from build123d import *

# Parameters (mm, degrees)
BOSS_EXTRUDE1_DEPTH           = 2.5
SKETCH2_W                     = 7
SKETCH2_H                     = 2.5
BOSS_EXTRUDE2_DEPTH           = 9.5
CUT_EXTRUDE1_DEPTH            = 9.5
SKETCH4_R                     = 1.275
CUT_EXTRUDE2_DEPTH            = 9.5
CBORE_FOR_M2_SHCS1_AT_2_COUNT = 2
CBORE_FOR_M2_SHCS1_AT_2_PITCH = 10
SKETCH8_R                     = 2.2
CUT_EXTRUDE3_DEPTH            = 9.5
SKETCH11_W                    = 19.05
SKETCH11_H                    = 19.05
BOSS_EXTRUDE3_DEPTH           = 5
FILLET1_R                     = 0.2


with BuildPart() as part:
    # Sketch1 → Boss-Extrude1 (new body, symmetric)
    with BuildSketch(Plane(origin=(0, 0, 0), x_dir=(1, 0, 0), z_dir=(0, 1, 0))):
        with BuildLine():
            Line((1.96, 0), (8, 0))
            ThreePointArc((8, 0), (0, -8), (-8, 0))
            Line((-8, 0), (-1.96, 0))
            ThreePointArc((-1.96, 0), (0, -1.96), (1.96, 0))
        make_face()
    extrude(amount=BOSS_EXTRUDE1_DEPTH, both=True)

    # Sketch2 → Boss-Extrude2 (add)
    with BuildSketch(Plane(origin=(0, 2.5, 0), x_dir=(1, 0, 0), z_dir=(0, 1, 0))):
        with Locations((0, -5)):
            Rectangle(SKETCH2_W, SKETCH2_H)
    extrude(amount=BOSS_EXTRUDE2_DEPTH)

    # Sketch3 → Cut-Extrude1 (cut)
    with BuildSketch(Plane(origin=(0, 0, 3.75), x_dir=(-1, 0, 0), z_dir=(0, 0, -1))):
        with BuildLine():
            Line((-3.5, 8.5), (-3.5, 14.886359519))
            Line((-3.5, 14.886359519), (0, 16.809201746))
            Line((0, 16.809201746), (3.5, 14.5))
            Line((3.5, 14.5), (3.5, 8.5))
            ThreePointArc((3.5, 8.5), (0, 12), (-3.5, 8.5))
        make_face()
    extrude(amount=-CUT_EXTRUDE1_DEPTH, mode=Mode.SUBTRACT)

    # Sketch4 → Cut-Extrude2 (cut)
    with BuildSketch(Plane(origin=(0, 0, 3.75), x_dir=(-1, 0, 0), z_dir=(0, 0, -1))):
        with Locations((0, 8.5)):
            Circle(SKETCH4_R)
    extrude(amount=-CUT_EXTRUDE2_DEPTH, mode=Mode.SUBTRACT)

    # Sketch7 → CBORE for M2 SHCS1 (revolve, cut)
    with BuildSketch(Plane(origin=(5, 0, 7), x_dir=(0, -1, 0), z_dir=(1, 0, 0))):
        Polygon((0, 0), (0, 7), (1.2, 7), (1.2, 2), (2.2, 2), (2.2, 0), align=None)
    cbore_for_m2_shcs1 = revolve(axis=Axis((5, 0, 13.35), (0, 0, -1)), mode=Mode.SUBTRACT)

    # CBORE for M2 SHCS1 at 2: CBORE for M2 SHCS1 ×2
    with Locations(*[(-i * CBORE_FOR_M2_SHCS1_AT_2_PITCH, 0, 0) for i in range(1, CBORE_FOR_M2_SHCS1_AT_2_COUNT)]):
        add(cbore_for_m2_shcs1, mode=Mode.SUBTRACT)

    # Sketch8 → Cut-Extrude3 (cut)
    with BuildSketch(Plane(origin=(0, 0, 7), x_dir=(-1, 0, 0), z_dir=(0, 0, -1))):
        with Locations((-5, 0)):
            Circle(SKETCH8_R)
        with Locations((5, 0)):
            Circle(SKETCH8_R)
    extrude(amount=-CUT_EXTRUDE3_DEPTH, mode=Mode.SUBTRACT)

    # Sketch11 → Boss-Extrude3 (add)
    with BuildSketch(Plane.XZ.offset(2.5)):
        with Locations((0, 4)):
            Rectangle(SKETCH11_W, SKETCH11_H)
    extrude(amount=BOSS_EXTRUDE3_DEPTH)

    # Fillet1
    fillet1_edges = [part.edges().sort_by_distance(p)[0] for p in [
        (1.96, 0, 0),
        (-1.96, 0, 0),
    ]]
    fillet(fillet1_edges, radius=FILLET1_R)


solid = part.part
Can you work these out from the model? Positions are in its coordinate system, mm. A direction names the side the tool comes from. Give positions to 0.01 mm unless a question says otherwise; leave off trailing zeros. Write each loop counter-clockwise with the first axis right and the second up, starting at its lowest first coordinate (ties: lowest second). Pieces come first, ordered by that corner, then holes. Notation, with made-up numbers: (-12.75, -24) -> (9.25, -24) arc R10 cw to (9.25, -15) -> close; hole circle Ø2 at (8, 82.5). An arc over 180 degrees is marked (long way). Answer as a JSON object with one key per item and string values. Group by question number.
Item 1: We'd pull the mould along X, two halves only. Please class faces 1 (the face through (-0.04, 0.04, 1.96)), 2 (the face through (-9.525, -5, 4)), 3 (the face through (0, -5, -5.525)): +X half, -X half, draft (parallel to the pull), parting line (faces both ways), or undercut.
Item 2: Please list where these lines run through material, in increasing order: line 1 (X direction, y = 0, z = 2.3); line 2 (X direction, y = 0, z = 3.85); line 3 (Y direction, x = 0.5, z = 6.5). Write a range as [from, to].
Item 3: Suppose I cut it at B-B (x = -5). Please give me the cut outline in (y, z) (3 decimals).
Item 4: Suppose I cut it at C-C (x = 0). Please give me the cut outline in (y, z) (3 decimals).
Item 5: For faces 4 (the face through (6, 1, 0)), 5 (the face through (0, 0, 8)), 6 (the face through (3.5, 5, 5)), 7 (the face through (-4, -1, 5)), which set-ups out of +Z, -Z, +X, -X, +Y, -Y let a thin tool reach every point of the face, with its end or its side?
Item 6: Suppose I cut it at D-D (z = 11.75). Please give me the cut outline in (x, y) (3 decimals).
Item 7: Suppose I cut it at A-A (y = 0). Please give me the cut outline in (x, z) (3 decimals), plus the area to 3 significant figures.
Item 8: I'm going to push flat-ended pins straight in: P1, Ø4, axis at y = 5.5, z = 5, coming from the +X side; P2, Ø1, axis at x = -4.5, y = -1, coming from the +Z side; P3, Ø4, axis at x = 4, z = 2.5, coming from the +Y side. Where does each tip first touch, or does it pass through?
Findings:
{
 "1": {"face 1": "undercut", "face 2": "-X half", "face 3": "draft"},
 "2": {"line 1": "x = [-7.66, -6.2], [-3.8, 3.8], [6.2, 7.66]", "line 2": "x = [-7.01, -6.2], [-3.8, 3.8], [6.2, 7.01]", "line 3": "y = [-7.5, 2.5]"},
 "3": {"outline": "(-7.5, -5.525) -> (-2.5, -5.525) -> (-2.5, 0) -> (-1.2, 0) -> (-1.2, 5) -> (-2.2, 5) -> (-2.2, 6.245) -> (-2.5, 6.245) -> (-2.5, 13.525) -> (-7.5, 13.525) -> close; (1.2, 0) -> (2.5, 0) -> (2.5, 6.245) -> (2.2, 6.245) -> (2.2, 5) -> (1.2, 5) -> close"},
 "4": {"outline": "(-7.5, -5.525) -> (-2.5, -5.525) -> (-2.5, 1.96) -> (2.5, 1.96) -> (2.5, 3.75) -> (7.225, 3.75) -> (7.225, 6.25) -> (2.5, 6.25) -> (2.5, 8) -> (-2.5, 8) -> (-2.5, 13.525) -> (-7.5, 13.525) -> close; (9.775, 3.75) -> (12, 3.75) -> (12, 6.25) -> (9.775, 6.25) -> close"},
 "5": {"face 4": "-Z, +X, -X, +Y", "face 5": "+Z, +Y", "face 6": "+Z, -Z, +X, +Y", "face 7": "+Z"},
 "6": {"outline": "(-9.525, -7.5) -> (9.525, -7.5) -> (9.525, -2.5) -> (-9.525, -2.5) -> close"},
 "7": {"outline": "(-8, 0) -> (-6.2, 0) -> (-6.2, 5) -> (-6.245, 5) arc R8 ccw to start; (-3.8, 0) -> (-2.151, 0) arc R0.2 ccw to (-1.952, 0.181) arc R1.96 cw to (1.952, 0.181) arc R0.2 ccw to (2.151, 0) -> (3.8, 0) -> (3.8, 5) -> (2.8, 5) -> (2.8, 7.494) arc R8 ccw to (-2.8, 7.494) -> (-2.8, 5) -> (-3.8, 5) -> close; (6.2, 0) -> (8, 0) arc R8 ccw to (6.245, 5) -> (6.2, 5) -> close", "area": "60.3 mm²"},
 "8": {"P1": "stops at x = 3.5", "P2": "stops at z = 5", "P3": "stops at y = 11.01"}
}
